from build123d import *

# Parameters (mm, degrees)
CROQUIS1_W                      = 275
CROQUIS1_H                      = 260
BRIDA_BASE1_DEPTH               = 6
CORTAR_EXTRUIR1_DEPTH           = 190.320495457
CORTAR_EXTRUIR2_DEPTH           = 190.320495457
CORTAR_EXTRUIR2_DEPTH_BACK      = 190.320495457
CROQUIS3_R                      = 1.875
RANURA_START                    = -6
RANURA_DE_MARGEN_PARA_M61_DEPTH = 6
CROQUIS8_R                      = 1.2
CORTAR_EXTRUIR4_DEPTH           = 190.320495457
TALADRO_DE_MARGEN_PARA_M31_D    = 3.4


# Read off the part's stored shape, not the designer's step: Ranura de margen para M61
# Sheet-metal steps are written as plain solids
with BuildPart() as part:
    # Croquis1 → Brida base1 (new body)
    with BuildSketch(Plane.XY):
        Rectangle(CROQUIS1_W, CROQUIS1_H)
    extrude(amount=-BRIDA_BASE1_DEPTH)

    # Croquis2 → Cortar-Extruir1 (cut, through all)
    with BuildSketch(Plane.XY):
        with BuildLine():
            Line((-101.5, 38.67), (29.25, 38.67))
            ThreePointArc((29.25, 38.67), (41.25, 50.67), (29.25, 62.67))
            Line((29.25, 62.67), (-101.5, 62.67))
            ThreePointArc((-101.5, 62.67), (-113.5, 50.67), (-101.5, 38.67))
        make_face()
    extrude(amount=-CORTAR_EXTRUIR1_DEPTH, mode=Mode.SUBTRACT)

    # Croquis3 → Cortar-Extruir2 (cut, two sides: drawn at the far end of the back side and taken through both)
    with BuildSketch(Plane.XY.offset(-CORTAR_EXTRUIR2_DEPTH_BACK)):
        with Locations((88, 84.63)):
            Circle(CROQUIS3_R)
        with Locations((88, 124.63)):
            Circle(CROQUIS3_R)
        with Locations((60, 124.63)):
            Circle(CROQUIS3_R)
    extrude(amount=CORTAR_EXTRUIR2_DEPTH + CORTAR_EXTRUIR2_DEPTH_BACK, mode=Mode.SUBTRACT)

    # Ranura de margen para M61 outline → Ranura de margen para M61 (cut)
    with BuildSketch(Plane.XY.offset(RANURA_START)):
        with BuildLine():
            Line((120, 125), (117, 125))
            ThreePointArc((117, 125), (113.5, 121.5), (117, 118))
            Line((117, 118), (120, 118))
            ThreePointArc((120, 118), (123.5, 121.5), (120, 125))
        make_face()
        with BuildLine():
            ThreePointArc((-120, 125), (-123.5, 121.5), (-120, 118))
            Line((-120, 118), (-117, 118))
            ThreePointArc((-117, 118), (-113.5, 121.5), (-117, 125))
            Line((-117, 125), (-120, 125))
        make_face()
        with BuildLine():
            Line((-117, -118), (-120, -118))
            ThreePointArc((-120, -118), (-123.5, -121.5), (-120, -125))
            Line((-120, -125), (-117, -125))
            ThreePointArc((-117, -125), (-113.5, -121.5), (-117, -118))
        make_face()
        with BuildLine():
            ThreePointArc((117, -118), (113.5, -121.5), (117, -125))
            Line((117, -125), (120, -125))
            ThreePointArc((120, -125), (123.5, -121.5), (120, -118))
            Line((120, -118), (117, -118))
        make_face()
    extrude(amount=RANURA_DE_MARGEN_PARA_M61_DEPTH, mode=Mode.SUBTRACT)

    # Croquis8 → Cortar-Extruir4 (cut, through all)
    with BuildSketch(Plane.XY):
        with Locations((5, -127.5)):
            Circle(CROQUIS8_R)
    extrude(amount=-CORTAR_EXTRUIR4_DEPTH, mode=Mode.SUBTRACT)

    # Taladro de margen para M31 (through all)
    with Locations(Plane(origin=(0, 0, -6), x_dir=(-1, 0, 0), z_dir=(0, 0, -1))):
        with Locations((10, 125), (-10, 125)):
            Hole(TALADRO_DE_MARGEN_PARA_M31_D / 2)


solid = part.part
Check sheet for the modelled part. Datum: model origin and axes. Units: mm. A direction names the side the tool comes from. Round coordinates to 2 decimals unless told otherwise and drop trailing zeros. Write each loop counter-clockwise with the first axis right and the second up, starting at its lowest first coordinate (ties: lowest second). Pieces come first, ordered by that corner, then holes. Notation, with made-up numbers: (20.5, 9) -> (40.5, 9) arc R27 ccw to (40.5, 30) -> close; hole circle Ø1 at (-37, 41). An arc over 180 degrees is marked (long way). Answer as CSV lines item,"result". Start each with the question number.
1) Section check C-C on x = -66.5. Enter the section's corners in (y, z).
2) Release check for a two-part mould opening along Y. For faces 3 (the flat face through (-2, 2, 0)), 4 (the flat face through (-2, 130, -3)), 5 (the cylindrical face through (-123.5, -121.4, -3)) record: pulls with the +Y half, pulls with the -Y half, needs draft (parallel to the pull), parting line crosses it, or undercut.
3) Tool access check on faces 1 (the flat face through (-2, 2, -6)), 2 (the cylindrical face through (123.5, -121.6, -3)). Record the directions out of +Z, -Z, +X, -X, +Y, -Y that give a thin tool (end or side, any length) a straight path to the whole face; none if there is none.
4) Section check B-B on z = -2.4. State how many separate pieces and enclosed holes the cut face has, and give its area (3 significant figures).
5) Section check A-A on y = 50.67. Enter the section's corners in (x, z).
6) Material ranges on line 1 (Y direction, x = 5, z = -1.25); line 2 (Y direction, x = -120.5, z = -4.2); line 3 (Y direction, x = 18.5, z = -1.7), recorded low to high. Write a range as from..to.
Found:
1,outline,"(-130, -6) -> (38.67, -6) -> (38.67, 0) -> (-130, 0) -> close; (62.67, -6) -> (130, -6) -> (130, 0) -> (62.67, 0) -> close"
2,face 3,"needs draft"
2,face 4,"pulls with the +Y half"
2,face 5,"undercut"
3,face 1,"-Z, +X, -X, +Y, -Y"
3,face 2,"+Z, -Z"
4,separate pieces,"1"
4,enclosed holes,"11"
4,area,"67,600 mm^2"
5,outline,"(-137.5, -6) -> (-113.5, -6) -> (-113.5, 0) -> (-137.5, 0) -> close; (41.25, -6) -> (137.5, -6) -> (137.5, 0) -> (41.25, 0) -> close"
6,line 1,"y = -130..-128.7, -126.3..38.67, 62.67..130"
6,line 2,"y = -130..-124.96, -118.04..118.04, 124.96..130"
6,line 3,"y = -130..38.67, 62.67..130"
